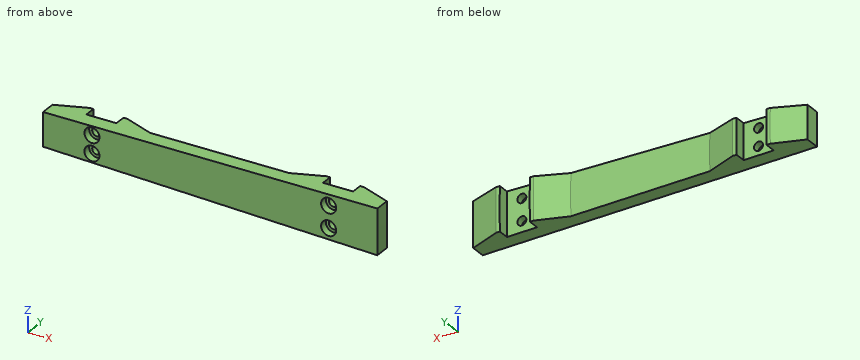
from build123d import *

# Parameters (mm, degrees)
EXTRUDE_1_DEPTH     = 2.5
SKETCH_5_R          = 0.6
CUT_EXTRUDE_1_DEPTH = 19.036421485
CUT_EXTRUDE_START   = -2
SKETCH_5_3_R        = 1
CUT_EXTRUDE_2_DEPTH = 1
REVOLVE_1_ANGLE     = 1
SKETCH_9_R          = 0.6
CUT_EXTRUDE_3_DEPTH = 41.426698916
SKETCH_9_3_R        = 1
CUT_EXTRUDE_4_DEPTH = 1
SKETCH_10_W         = 44.5
SKETCH_10_H         = 2.5
CUT_EXTRUDE_5_DEPTH = 41.528606999


with BuildPart() as part:
    # 草图4 → 凸台-拉伸1 (new body)
    with BuildSketch(Plane.XY):
        Polygon((8.5, -1.5), (17.75, -1.5), (17.75, -3.5), (-4.5, -3.5), (-4.5, -1.5), (-0.5, 0), (0, 0), (0, -1.5), (4, -1.5), (4, 0), (4.5, 0), align=None)
    extrude(amount=EXTRUDE_1_DEPTH)

    # 草图5 → 切除-拉伸1 (cut, through all)
    with BuildSketch(Plane(origin=(0, -1.5, 0), x_dir=(1, 0, 0), z_dir=(0, 1, 0))):
        with Locations(Location((2, -1.25, 0), (0, 0, 270))):
            Circle(SKETCH_5_R)
    extrude(amount=-CUT_EXTRUDE_1_DEPTH, mode=Mode.SUBTRACT)

    # 草图5<3> → 切除-拉伸2 (cut)
    with BuildSketch(Plane(origin=(0, -1.5, 0), x_dir=(1, 0, 0), z_dir=(0, 1, 0)).offset(CUT_EXTRUDE_START)):
        with Locations((2, -1.25)):
            Circle(SKETCH_5_3_R)
    extrude(amount=CUT_EXTRUDE_2_DEPTH, mode=Mode.SUBTRACT)

    # 镜向1: part across plane


with BuildPart() as part_1:
    add(part.part)
    add(part.part.mirror(Plane(origin=(17.75, 0, 2.5), x_dir=(0, 0, 1), z_dir=(1, 0, 0))))

    # 草图6 → 旋转1 (revolve)
    with BuildSketch(Plane.XY.offset(2.5)):
        Polygon((0, 0), (-0.5, 0), (-4.5, -1.5), (-4.5, -3.5), (40, -3.5), (40, -1.5), (36, 0), (35.5, 0), (35.5, -1.5), (31.5, -1.5), (31.5, 0), (31, 0), (27, -1.5), (8.5, -1.5), (4.5, 0), (4, 0), (4, -1.5), (0, -1.5), align=None)
    revolve(axis=Axis((-132.25, 94.8535776, 2.5), (0, -1, 0)), revolution_arc=REVOLVE_1_ANGLE)

    # 草图9 → 切除-拉伸3 (cut, through all)
    with BuildSketch(Plane(origin=(0, -1.5, 0), x_dir=(1, 0, 0), z_dir=(0, 1, 0))):
        with Locations(Location((1.994888171, -3.671537391, 0), (0, 0, 180))):
            Circle(SKETCH_9_R)
        with Locations(Location((33.493688748, -3.946423259, 0), (0, 0, 180))):
            Circle(SKETCH_9_R)
    extrude(amount=-CUT_EXTRUDE_3_DEPTH, mode=Mode.SUBTRACT)

    # 草图9<3> → 切除-拉伸4 (cut)
    with BuildSketch(Plane(origin=(0, -1.5, 0), x_dir=(1, 0, 0), z_dir=(0, 1, 0)).offset(CUT_EXTRUDE_START)):
        with Locations((1.994888171, -3.671537391)):
            Circle(SKETCH_9_3_R)
        with Locations((33.493688748, -3.946423259)):
            Circle(SKETCH_9_3_R)
    extrude(amount=CUT_EXTRUDE_4_DEPTH, mode=Mode.SUBTRACT)

    # 草图10 → 切除-拉伸5 (cut, through all)
    with BuildSketch(Plane(origin=(0, 0, 0), x_dir=(1, 0, 0), z_dir=(0, 1, 0))):
        with Locations((17.75, -1.25)):
            Rectangle(SKETCH_10_W, SKETCH_10_H)
    extrude(amount=-CUT_EXTRUDE_5_DEPTH, mode=Mode.SUBTRACT)

    # 镜向2: part across plane


with BuildPart() as part_2:
    add(part_1.part)
    add(part_1.part.mirror(Plane(origin=(40, -3.5, 2.5), x_dir=(1, 0, 0), z_dir=(0, 0, 1))))


solid = part_2.part
Here's how the part is built. I have some questions about the finished solid (model axes, mm). Coordinates: 2 decimals unless noted, no trailing zeros. Write each loop counter-clockwise with the first axis right and the second up, starting at its lowest first coordinate (ties: lowest second). Pieces come first, ordered by that corner, then holes.
Item 1: I want a section at B-B on y = -3. Write out the boundary of the cut face in (x, z), and give its area (3 significant figures).
Item 2: If I drill on line 1 (X direction, y = -1.7, z = 1.5); line 2 (X direction, y = -1.8, z = 3.75); line 3 (Y direction, x = 12.5, z = 3.5), over which ranges is the centre line in solid material (lowest first)?
Item 3: I want a section at C-C on x = 14. Write out the boundary of the cut face in (y, z), and give its area (3 significant figures).
Item 4: I want a section at A-A on y = -0.85. Write out the boundary of the cut face in (x, z), and give its area (3 significant figures).
Item 5: Will these pins go through, and if not, where does the flat tip stop? pin 1 (1.5 mm diameter, centred on y = -1.5, z = 1, fed in from +X); pin 2 (2 mm diameter, centred on x = 22, y = -3, fed in from -Z); pin 3 (1.6 mm diameter, centred on x = 1.99, z = 3.67, fed in from +Y).
Item 6: I want a section at D-D on x = 26.5. Write out the boundary of the cut face in (y, z), and give its area (3 significant figures).
Findings below:
1. outline: (-4.52, 0.27) - (39.97, -0.51) arc R172.25 ccw to (39.97, 5.51) - (-4.52, 4.73) arc R127.75 cw to start; hole circle Ø2 at (1.99, 1.33); hole circle Ø2 at (1.99, 3.67); hole circle Ø2 at (33.49, 1.05); hole circle Ø2 at (33.49, 3.95)
1. area: 220 mm2
2. line 1: x = -4.5 to 1.42, 2.57 to 33.09, 33.89 to 40
2. line 2: x = -4.51 to 1.4, 2.59 to 32.93, 34.06 to 40
2. line 3: y = -3.5 to -1.5
3. outline: (-3.5, -0.05) - (-1.5, -0.05) - (-1.5, 5.05) - (-3.5, 5.05) - close
3. area: 10.2 mm2
4. outline: (-2.79, 0.24) - (-0.02, 0.19) arc R132.25 ccw to (-0.02, 4.81) - (-2.79, 4.76) arc R129.48 cw to start; (3.98, 0.12) - (6.75, 0.07) arc R139.02 ccw to (6.75, 4.93) - (3.98, 4.88) arc R136.25 cw to start; (28.71, -0.31) - (31.48, -0.36) arc R163.75 ccw to (31.48, 5.36) - (28.71, 5.31) arc R160.98 cw to start; (35.47, -0.43) - (38.24, -0.48) arc R170.52 ccw to (38.24, 5.48) - (35.47, 5.43) arc R167.75 cw to start
4. area: 57.9 mm2
5. pin 1: stops at x = 40
5. pin 2: stops at z = -0.21
5. pin 3: stops at y = -1.5
6. outline: (-3.5, -0.27) - (-1.5, -0.27) - (-1.5, 5.27) - (-3.5, 5.27) - close
6. area: 11.1 mm2
